from build123d import *

# Parameters (mm, degrees)
EXTRUDE_1_DEPTH     = 21
SKETCH_2_W          = 15.5
SKETCH_2_H          = 12
EXTRUDE_2_DEPTH     = 18.5
SKETCH_4_R          = 1.75
CUT_EXTRUDE_2_DEPTH = 41.883982194
SKETCH_5_R          = 1.75
CUT_EXTRUDE_3_DEPTH = 41.883982194
SKETCH_6_R          = 1.75
CUT_EXTRUDE_4_DEPTH = 40.54111784
FILLET_1_R          = 9


with BuildPart() as part:
    # ｽｹｯﾁ1 → ﾎﾞｽ - 押し出し1 (new body)
    with BuildSketch(Plane(origin=(0, 0, 0), x_dir=(1, 0, 0), z_dir=(0, 1, 0))):
        Polygon((0, 18.5), (0, 0), (15.5, 0), (15.5, 4), (4, 4), (4, 14.5), (15.5, 14.5), (15.5, 18.5), align=None)
    extrude(amount=EXTRUDE_1_DEPTH)

    # ｽｹｯﾁ2 → ﾎﾞｽ - 押し出し2 (add)
    with BuildSketch(Plane.XY):
        with Locations((7.75, 27)):
            Rectangle(SKETCH_2_W, SKETCH_2_H)
    extrude(amount=-EXTRUDE_2_DEPTH)

    # ｽｹｯﾁ4 → ｶｯﾄ - 押し出し2 (cut, through all)
    with BuildSketch(Plane.XY):
        with Locations((9.5, 15)):
            Circle(SKETCH_4_R)
    extrude(amount=-CUT_EXTRUDE_2_DEPTH, mode=Mode.SUBTRACT)

    # ｽｹｯﾁ5 → ｶｯﾄ - 押し出し3 (cut, through all)
    with BuildSketch(Plane.ZY):
        with Locations((-9.25, 27)):
            Circle(SKETCH_5_R)
    extrude(amount=-CUT_EXTRUDE_3_DEPTH, mode=Mode.SUBTRACT)

    # ｽｹｯﾁ6 → ｶｯﾄ - 押し出し4 (cut, through all)
    with BuildSketch(Plane(origin=(4, 0, 0), x_dir=(0, 0, -1), z_dir=(1, 0, 0))):
        with Locations((9.25, 5)):
            Circle(SKETCH_6_R)
    extrude(amount=-CUT_EXTRUDE_4_DEPTH, mode=Mode.SUBTRACT)

    # ﾌｨﾚｯﾄ1
    fillet_1_edges = [part.edges().sort_by_distance(p)[0] for p in [
        (7.75, 33, -18.5),
        (7.75, 33, 0),
    ]]
    fillet(fillet_1_edges, radius=FILLET_1_R)


solid = part.part
The listing builds one solid part. Answer for the finished solid, in the listing's coordinates (mm). A direction names the side the tool comes from. Round coordinates to 2 decimals unless told otherwise and drop trailing zeros. Loops run counter-clockwise (first coordinate to the right, second up) from the corner with the lowest first, then second, coordinate; pieces in that order, holes last. Notation, with made-up numbers: M 7,38.5 L 61,38.5 A21 cw 61,58.5 Z; hole C -36,33.25 d4. An arc over 180 degrees is marked long. Write each question's results on one line, items separated by ' | '. Start each with the question number.
1) Find section A-A on x = 9.5. Write down the section's boundary in (y, z).
2) Find section C-C on x = 13.75. Write down the section's boundary in (y, z).
3) Each of these flat-tipped pins is pushed along its axis until it touches: pin 1 (4 mm diameter, centred on y = 5, z = -9.25, fed in from +X); pin 2 (2 mm diameter, centred on x = 9, z = -16.5, fed in from +Y); pin 3 (5 mm diameter, centred on x = 8, z = -11.5, fed in from -Y); pin 4 (2 mm diameter, centred on x = 9.5, y = 15, fed in from -Z). Where does it stop, or does it pass through?
4) Find section B-B on y = 15. Write down the section's boundary in (x, z), plus the area to 3 significant figures.
5) Determine the mould class of faces 3 (the cylindrical face through (7.642, 28.476, -8.309)), 4 (the flat face through (10, 21, -9)), 5 (the flat face through (8, 12, -18.5)), 6 (the cylindrical face through (9.272, 16.735, -16.472)) for opening direction Y: pulls with the +Y half, pulls with the -Y half, needs draft (parallel to the pull), parting line crosses it, or undercut.
6) Which of the six approach directions +Z, -Z, +X, -X, +Y, -Y give full straight-line access (tool end or side, diameter ignored) to faces 1 (the flat face through (4, 10, -9)), 2 (the cylindrical face through (7.858, 30.434, -2.706))?
7) Straight lines are drawn through the part: probe 1 along Y at (x, z) = (2.45, -9.25); probe 2 along Z at (x, y) = (12.25, 20.5); probe 3 along X at (y, z) = (3, -10.25). For each, find the intervals that lie inside material, in ascending order.
8) Find section D-D on y = 26.5. Write down the section's boundary in (x, z).
Final values:
1) outline: M 0,-18.5 L 13.25,-18.5 L 13.25,-14.5 L 0,-14.5 Z; M 0,-4 L 13.25,-4 L 13.25,0 L 0,0 Z; M 16.75,-18.5 L 24,-18.5 A9 ccw 33,-9.5 L 33,-9 A9 ccw 24,0 L 16.75,0 L 16.75,-4 L 21,-4 L 21,-14.5 L 16.75,-14.5 Z; hole C 27,-9.25 d3.5
2) outline: M 0,-18.5 L 24,-18.5 A9 ccw 33,-9.5 L 33,-9 A9 ccw 24,0 L 0,0 L 0,-4 L 21,-4 L 21,-14.5 L 0,-14.5 Z; hole C 27,-9.25 d3.5
3) pin 1: x = 4 | pin 2: y = 30.71 | pin 3: y = 21 | pin 4: through
4) outline: M 0,-18.5 L 7.75,-18.5 L 7.75,-14.5 L 4,-14.5 L 4,-4 L 7.75,-4 L 7.75,0 L 0,0 Z; M 11.25,-18.5 L 15.5,-18.5 L 15.5,-14.5 L 11.25,-14.5 Z; M 11.25,-4 L 15.5,-4 L 15.5,0 L 11.25,0 Z | area: 138 mm²
5) face 3: undercut | face 4: pulls with the -Y half | face 5: needs draft | face 6: undercut
6) face 1: +X, -Y | face 2: +Z, +X, -X, +Y
7) probe 1: 0 to 3.25, 6.75 to 25.25, 28.75 to 33 | probe 2: -18.5 to -14.5, -4 to 0 | probe 3: 0 to 4
8) outline: M 0,-18.15 L 15.5,-18.15 L 15.5,-10.93 L 0,-10.93 Z; M 0,-7.57 L 15.5,-7.57 L 15.5,-0.35 L 0,-0.35 Z
